For this review, use the dimensioned drawing (mm, ordinates from the lowest corner) and the shaded views. A direction names the side the tool comes from. Coordinates: 2 decimals unless noted, no trailing zeros. Loops run counter-clockwise (first coordinate to the right, second up) from the corner with the lowest first, then second, coordinate; pieces in that order, holes last. Notation, with made-up numbers: M 79,27.5 L 96,27.5 A29 cw 96,60.5 Z; hole C 22,-28.5 d2. An arc over 180 degrees is marked long. One line per item, written item: value.
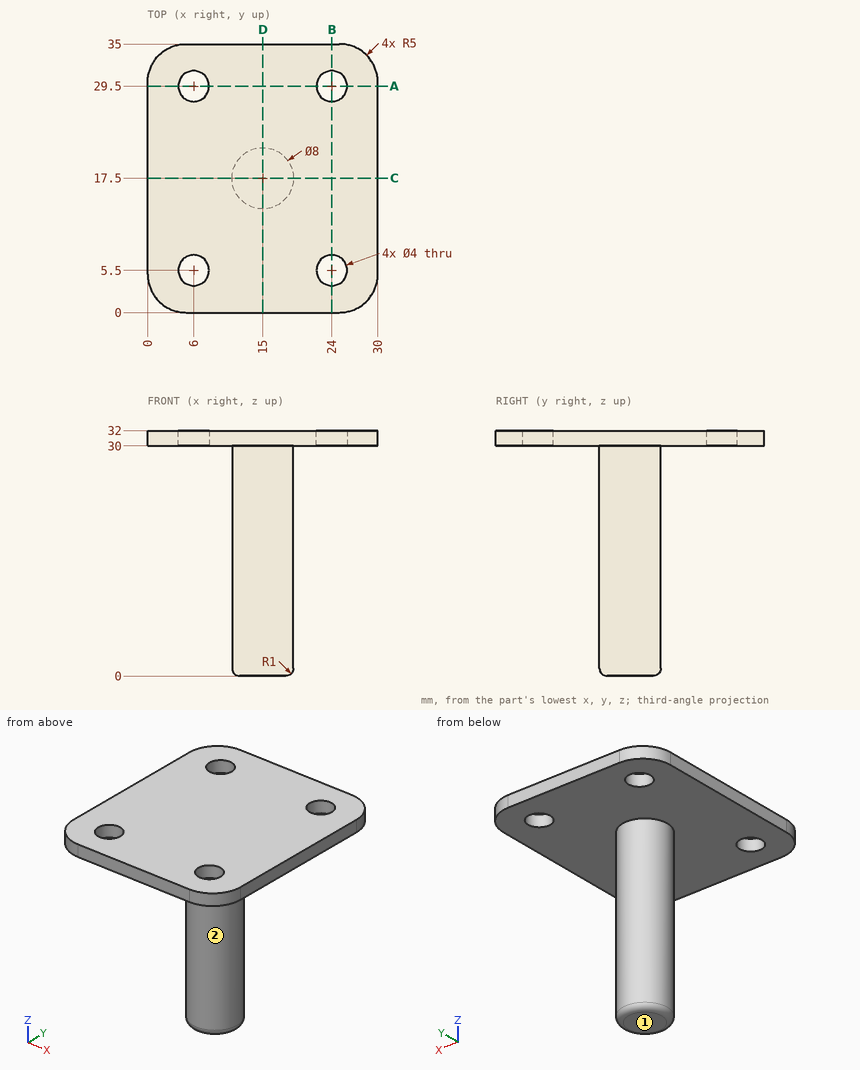
(1) Tool access review of the marked faces 1 and 2: name each direction out of +Z, -Z, +X, -X, +Y, -Y from which nothing blocks a thin tool from reaching the whole face with its end or side.
Reply:
face 1: -Z, +X, -X, +Y, -Y
face 2: -Z
(2) We need section B-B on x = 24. State the section outline as (y, z) points.
Reply:
outline: M 0,30 L 3.5,30 L 3.5,32 L 0,32 Z; M 7.5,30 L 27.5,30 L 27.5,32 L 7.5,32 Z; M 31.5,30 L 35,30 L 35,32 L 31.5,32 Z
(3) We need section C-C on y = 17.5. State the section outline as (x, z) points.
Reply:
outline: M 0,30 L 11,30 L 11,1 A1 ccw 12,0 L 18,0 A1 ccw 19,1 L 19,30 L 30,30 L 30,32 L 0,32 Z
(4) To check wall thickness, follow line 1 along Y through (x, z) = (24, 31.3); line 2 along Z through (x, y) = (5.25, 26); line 3 along Y through (x, z) = (13.75, 29.5). State the ranges of each line that lie inside material, in increasing order. Write a range as [from, to].
Reply:
line 1: y = [0, 3.5], [7.5, 27.5], [31.5, 35]
line 2: z = [30, 32]
line 3: y = [13.7, 21.3]
(5) We need section D-D on x = 15. State the section outline as (y, z) points, then the cut area to 3 significant figures.
Reply:
outline: M 0,30 L 13.5,30 L 13.5,1 A1 ccw 14.5,0 L 20.5,0 A1 ccw 21.5,1 L 21.5,30 L 35,30 L 35,32 L 0,32 Z
area: 310 mm2
(6) Insertion check: pin 1 (6 mm diameter, centred on x = 26, y = 15.5, fed in from -Z); pin 2 (5 mm diameter, centred on y = 15, z = 22, fed in from +X); pin 3 (6 mm diameter, centred on x = 10.5, z = 16, fed in from -Y); pin 4 (12 mm diameter, centred on y = 28.5, z = 7.5, fed in from -X). Each pin has a flat end and moves straight along its axis. Give the tip position at first contact, or say it passes through.
Reply:
pin 1: stops at z = 30
pin 2: stops at x = 19
pin 3: stops at y = 13.79
pin 4: passes through
(7) We need section A-A on y = 29.5. State the section outline as (x, z) points, then the cut area to 3 significant figures.
Reply:
outline: M 0,30 L 4,30 L 4,32 L 0,32 Z; M 8,30 L 22,30 L 22,32 L 8,32 Z; M 26,30 L 30,30 L 30,32 L 26,32 Z
area: 44.0 mm2
